Here's how the part is built. I have some questions about the finished solid (model axes, mm). Face numbers are marked on the shaded views. Round coordinates to 2 decimals unless told otherwise and drop trailing zeros. Write each loop counter-clockwise with the first axis right and the second up, starting at its lowest first coordinate (ties: lowest second). Pieces come first, ordered by that corner, then holes. Notation, with made-up numbers: (-3, -19.5) -> (22, -19.5) arc R20 cw to (22, -10.5) -> close; hole circle Ø2 at (-14.5, -14.75). An arc over 180 degrees is marked (long way). Answer as CSV lines item,"result".
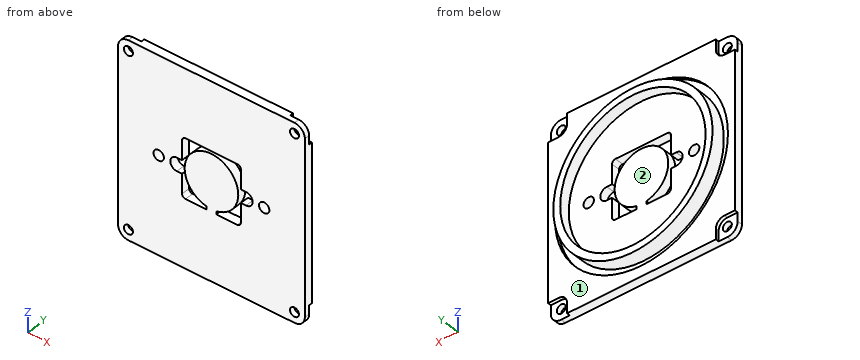
Autodesk Inventor part; units mm, degrees
ref_plane "YZ Plane" through (0, 0, 0) normal (1, 0, 0) x (0, 1, 0)
ref_plane "XZ Plane" through (0, 0, 0) normal (0, 1, 0) x (-1, 0, 0)
ref_plane "XY Plane" through (0, 0, 0) normal (0, 0, 1) x (1, 0, 0)
ref_plane "作業平面1" through (56.3598, -66.4332, -0.2999) normal (0, 1, 0) x (1, 0, 0)
sketch "スケッチ1" plane through (56.3598, -66.4332, -0.2999) normal (0, 1, 0) x (1, 0, 0)
  line L0 (9.655, 16.755) -> (9.655, 15.8775)
  arc A0 (6.855, 15.8775) -> (9.655, 15.8775) centre (8.255, 8.255) ccw
  line L1 (6.855, 15.8775) -> (6.855, 16.755)
  line L2 (6.855, 16.755) -> (0.755, 16.755)
  arc A1 (0.755, 16.755) -> (-0.245, 15.755) centre (0.755, 15.755) ccw
  line L3 (-0.245, 15.755) -> (-0.245, 10.155)
  line L4 (-0.245, 10.155) -> (-1.745, 10.155)
  arc A2 (-1.745, 10.155) -> (-1.745, 6.355) centre (-1.745, 8.255) ccw
  line L5 (-1.745, 6.355) -> (-0.245, 6.355)
  line L6 (-0.245, 6.355) -> (-0.245, 0.755)
  arc A3 (-0.245, 0.755) -> (0.755, -0.245) centre (0.755, 0.755) ccw
  line L7 (0.755, -0.245) -> (15.755, -0.245)
  arc A4 (15.755, -0.245) -> (16.755, 0.755) centre (15.755, 0.755) ccw
  line L8 (16.755, 0.755) -> (16.755, 6.355)
  line L9 (16.755, 6.355) -> (18.255, 6.355)
  arc A5 (18.255, 6.355) -> (18.255, 10.155) centre (18.255, 8.255) ccw
  line L10 (18.255, 10.155) -> (16.755, 10.155)
  line L11 (16.755, 10.155) -> (16.755, 15.755)
  arc A6 (16.755, 15.755) -> (15.755, 16.755) centre (15.755, 15.755) ccw
  line L12 (15.755, 16.755) -> (9.655, 16.755)
  circle A7 centre (-1.745, 8.255) radius 0.9
  circle A8 centre (18.255, 8.255) radius 0.9
  circle A9 centre (-6.985, 8.255) radius 1.5
  circle A10 centre (23.495, 8.255) radius 1.5
  line L13 (-15.745, -19.745) -> (32.255, -19.745)
  line L14 (35.255, -16.745) -> (35.255, 33.255)
  line L15 (32.255, 36.255) -> (-15.745, 36.255)
  line L16 (-18.745, 33.255) -> (-18.745, -16.745)
  line L17 (-18.745, -19.745) -> (35.255, 36.255) construction
  line L18 (35.255, -19.745) -> (-18.745, 36.255) construction
  line L19 (8.255, 36.255) -> (8.255, -19.745) construction
  line L20 (-18.745, 8.255) -> (35.255, 8.255) construction
  arc A11 (-15.745, 36.255) -> (-18.745, 33.255) centre (-15.745, 33.255) ccw
  arc A12 (35.255, 33.255) -> (32.255, 36.255) centre (32.255, 33.255) ccw
  arc A13 (32.255, -19.745) -> (35.255, -16.745) centre (32.255, -16.745) ccw
  arc A14 (-18.745, -16.745) -> (-15.745, -19.745) centre (-15.745, -16.745) ccw
  circle A15 centre (-15.745, 33.255) radius 1.3
  circle A16 centre (32.255, 33.255) radius 1.3
  circle A17 centre (-15.745, -16.745) radius 1.3
  circle A18 centre (32.255, -16.745) radius 1.3
  circle A19 centre (8.255, 8.255) radius 25
  line L21 (32.255, -16.745) -> (-15.745, -16.745) construction
  line L22 (-15.745, -16.745) -> (-15.745, 33.255) construction
  line L23 (-15.745, 33.255) -> (32.255, 33.255) construction
  line L24 (32.255, 33.255) -> (32.255, -16.745) construction
  line L25 (32.255, -16.745) -> (-15.745, 33.255) construction
  line L26 (-15.745, -16.745) -> (32.255, 33.255) construction
  point P0 (-56.3598, -0.2999)
  dimension "d0" = 3
  dimension "d2" = 54
  dimension "d3" = 2.6
  dimension "d4" = 50
  dimension "d7" = 48
  dimension "d8" = 50
  dimension "d9" = 56
extrude "押し出し1" add sketch "スケッチ1" along normal blind 2.5 contours A14 L16 A11 L15 A12 L14 A13 L13 | A19
sketch "スケッチ2" plane through (56.3598, -63.9332, -0.2999) normal (0, 1, 0) x (1, 0, 0)
  arc A0 (32.255, -19.745) -> (35.255, -16.745) centre (32.255, -16.745) ccw
  line L0 (35.255, -16.745) -> (35.255, 33.255)
  arc A1 (35.255, 33.255) -> (32.255, 36.255) centre (32.255, 33.255) ccw
  line L1 (32.255, 36.255) -> (-15.745, 36.255)
  arc A2 (-15.745, 36.255) -> (-18.745, 33.255) centre (-15.745, 33.255) ccw
  line L2 (-18.745, 33.255) -> (-18.745, -16.745)
  arc A3 (-18.745, -16.745) -> (-15.745, -19.745) centre (-15.745, -16.745) ccw
  line L3 (-15.745, -19.745) -> (32.255, -19.745)
  arc A4 (6.855, 15.8775) -> (9.655, 15.8775) centre (8.255, 8.255) ccw
  line L4 (9.655, 15.8775) -> (9.655, 16.755)
  line L5 (9.655, 16.755) -> (15.755, 16.755)
  arc A5 (16.755, 15.755) -> (15.755, 16.755) centre (15.755, 15.755) ccw
  line L6 (16.755, 15.755) -> (16.755, 10.155)
  line L7 (16.755, 10.155) -> (18.255, 10.155)
  arc A6 (18.255, 6.355) -> (18.255, 10.155) centre (18.255, 8.255) ccw
  line L8 (18.255, 6.355) -> (16.755, 6.355)
  line L9 (16.755, 6.355) -> (16.755, 0.755)
  arc A7 (15.755, -0.245) -> (16.755, 0.755) centre (15.755, 0.755) ccw
  line L10 (15.755, -0.245) -> (0.755, -0.245)
  arc A8 (-0.245, 0.755) -> (0.755, -0.245) centre (0.755, 0.755) ccw
  line L11 (-0.245, 0.755) -> (-0.245, 6.355)
  line L12 (-0.245, 6.355) -> (-1.745, 6.355)
  arc A9 (-1.745, 10.155) -> (-1.745, 6.355) centre (-1.745, 8.255) ccw
  line L13 (-1.745, 10.155) -> (-0.245, 10.155)
  line L14 (-0.245, 10.155) -> (-0.245, 15.755)
  arc A10 (0.755, 16.755) -> (-0.245, 15.755) centre (0.755, 15.755) ccw
  line L15 (0.755, 16.755) -> (6.855, 16.755)
  line L16 (6.855, 16.755) -> (6.855, 15.8775)
  circle A11 centre (-6.985, 8.255) radius 1.5
  circle A12 centre (23.495, 8.255) radius 1.5
  circle A13 centre (32.255, -16.745) radius 1.3
  circle A14 centre (-15.745, -16.745) radius 1.3
  circle A15 centre (32.255, 33.255) radius 1.3
  circle A16 centre (-15.745, 33.255) radius 1.3
  circle A17 centre (8.255, 8.255) radius 23
  circle A18 centre (8.255, 8.255) radius 21
  circle A19 centre (8.255, 8.255) radius 25
  arc A20 (-13.245, -16.745) -> (-15.745, -14.245) centre (-15.745, -16.745) ccw
  arc A21 (-15.745, 30.755) -> (-13.245, 33.255) centre (-15.745, 33.255) ccw
  arc A22 (32.255, -14.245) -> (29.755, -16.745) centre (32.255, -16.745) ccw
  arc A23 (29.755, 33.255) -> (32.255, 30.755) centre (32.255, 33.255) ccw
  line L17 (-15.745, -14.245) -> (-18.745, -14.245)
  line L18 (-13.245, -16.745) -> (-13.245, -19.745)
  line L19 (-15.745, 30.755) -> (-18.745, 30.755)
  line L20 (-13.245, 33.255) -> (-13.245, 36.255)
  line L21 (29.755, 33.255) -> (29.755, 36.255)
  line L22 (32.255, 30.755) -> (35.255, 30.755)
  line L23 (32.255, -14.245) -> (35.255, -14.245)
  line L24 (29.755, -16.745) -> (29.755, -19.745)
  line L25 (-18.745, 33.255) -> (-18.745, -16.745)
  line L26 (-15.745, -19.745) -> (32.255, -19.745)
  line L27 (32.255, 36.255) -> (-15.745, 36.255)
  line L28 (35.255, -16.745) -> (35.255, 33.255)
  point P0 (-56.3598, -0.2999)
  dimension "d10" = 46
  dimension "d11" = 2
  dimension "d14" = 50
  dimension "d15" = 2.5
extrude "押し出し2" add sketch "スケッチ2" along normal blind 3 contours A17
extrude "押し出し4" cut sketch "スケッチ2" against normal blind 1 contours L3 L24 A22 L23 L0 A0 | L3 A3 L2 L17 A20 L18 | L22 A23 L21 L1 A1 L0 | L2 A2 L1 L20 A21 L19 | A19
properties part number "Camera_Mount"
1. Suppose I cut it at A-A on x = 50. Please give me the cut outline in (y, z).
Numbers:
outline,"(-66.43, -36.55) -> (-63.93, -36.55) -> (-63.93, -28.84) -> (-64.93, -28.84) -> (-64.93, -26.31) -> (-60.93, -26.31) -> (-60.93, -23.63) -> (-63.93, -23.63) -> (-63.93, -9.92) -> (-66.43, -9.92) -> close; (-66.43, -7.19) -> (-63.93, -7.19) -> (-63.93, 6.53) -> (-60.93, 6.53) -> (-60.93, 9.2) -> (-64.93, 9.2) -> (-64.93, 11.73) -> (-63.93, 11.73) -> (-63.93, 19.45) -> (-66.43, 19.45) -> close"
2. Suppose I cut it at D-D on y = -65.8. Count the separate pieces of the cut face and the enclosed holes in it, and give its area (3 significant figures).
Numbers:
separate pieces,"1"
enclosed holes,"7"
area,"2,860 mm^2"
3. Suppose I cut it at C-C on x = 68.5. Please give me the cut outline in (y, z).
Numbers:
outline,"(-66.43, -36.55) -> (-63.93, -36.55) -> (-63.93, -33.25) -> (-64.93, -33.25) -> (-64.93, -31.22) -> (-60.93, -31.22) -> (-60.93, -29.19) -> (-63.93, -29.19) -> (-63.93, -17.05) -> (-66.43, -17.05) -> close; (-66.43, -15.26) -> (-63.93, -15.26) -> (-63.93, -1.85) -> (-66.43, -1.85) -> close; (-66.43, -0.05) -> (-63.93, -0.05) -> (-63.93, 12.08) -> (-60.93, 12.08) -> (-60.93, 14.11) -> (-64.93, 14.11) -> (-64.93, 16.14) -> (-63.93, 16.14) -> (-63.93, 19.45) -> (-66.43, 19.45) -> close"
4. If I drill on line 1 (Z direction, x = 58.5, y = -65.3); line 2 (Z direction, x = 46, y = -64.05); line 3 (X direction, y = -64.35, z = 1), over which ranges is the centre line in solid material (lowest first)?
Numbers:
line 1,"z = -36.55 to -17.05, -13.32 to -3.79, -0.05 to 19.45"
line 2,"z = -36.55 to -25.24, -22.06 to 4.95, 8.13 to 19.45"
line 3,"x = 37.61 to 41.51, 43.69 to 85.54, 87.72 to 91.61"
5. If we mould it in two halves opening along Z, with no side actions, what happens to the marked faces 1 and 2? For each: released by +Z, released by -Z, zero draft, split by the parting line, or undercut.
Numbers:
face 1,"zero draft"
face 2,"undercut"
6. For pin 1 Ø6 at (x, z) = (41.5, 15.5) entering from +Y; pin 2 Ø1.5 at (x, y) = (74, -62.5) entering from -Z; pin 3 Ø2.5 at (x, z) = (79.85, -8.55) entering from +Y; pin 4 Ø4.5 at (x, z) = (40.5, -34) entering from +Y, each with a flat end and sliding along its axis, tell me the tip position at first contact or that it passes through.
Numbers:
pin 1,"stops at y = -63.93"
pin 2,"stops at z = -29.87"
pin 3,"passes through"
pin 4,"stops at y = -64.93"
7. Suppose I cut it at B-B on z = -2.5. Please give me the cut outline in (x, y).
Numbers:
outline,"(37.61, -66.43) -> (56.11, -66.43) -> (56.11, -63.93) -> (44.51, -63.93) -> (44.51, -60.93) -> (42.43, -60.93) -> (42.43, -64.93) -> (40.36, -64.93) -> (40.36, -63.93) -> (37.61, -63.93) -> close; (59.78, -66.43) -> (69.45, -66.43) -> (69.45, -63.93) -> (59.78, -63.93) -> close; (73.11, -66.43) -> (91.61, -66.43) -> (91.61, -63.93) -> (88.87, -63.93) -> (88.87, -64.93) -> (86.8, -64.93) -> (86.8, -60.93) -> (84.72, -60.93) -> (84.72, -63.93) -> (73.11, -63.93) -> close"
